For this review, take the finished solid that the model builds, in its own axes (mm). Coordinates: 2 decimals unless noted, no trailing zeros. Write each loop counter-clockwise with the first axis right and the second up, starting at its lowest first coordinate (ties: lowest second). Pieces come first, ordered by that corner, then holes. Notation, with made-up numbers: M 59,79.5 L 87,79.5 A19 ccw 87,109.5 Z; hole C 52,-28.75 d11. An arc over 180 degrees is marked long. One line per question, with ' | ' between items.
from build123d import *

# Parameters (mm, degrees)
SKETCH3_R           = 1.016
SKETCH3_R_2         = 0.75
BOSS_EXTRUDE1_DEPTH = 3


with BuildPart() as part:
    # Sketch3 → Boss-Extrude1 (new body)
    with BuildSketch(Plane.XY):
        with BuildLine():
            Line((9.525, -8.382), (41.275, -8.382))
            ThreePointArc((41.275, -8.382), (60.325, 10.668), (41.275, 29.718))
            Line((41.275, 29.718), (9.525, 29.718))
            ThreePointArc((9.525, 29.718), (-9.525, 10.668), (9.525, -8.382))
        make_face()
        with Locations((57.15, 10.668)):
            Circle(SKETCH3_R, mode=Mode.SUBTRACT)
        with Locations((-6.35, 10.668)):
            Circle(SKETCH3_R, mode=Mode.SUBTRACT)
        with Locations((2.032, 22.606)):
            Circle(SKETCH3_R_2, mode=Mode.SUBTRACT)
        with Locations((2.032, -1.27)):
            Circle(SKETCH3_R_2, mode=Mode.SUBTRACT)
        with Locations((49.022, -1.27)):
            Circle(SKETCH3_R_2, mode=Mode.SUBTRACT)
        with Locations((49.022, 22.606)):
            Circle(SKETCH3_R_2, mode=Mode.SUBTRACT)
        Polygon((18.5674, 24.638), (32.2326, 24.638), (32.2326, 21.59), (51.054, 21.59), (51.054, -0.254), (-0.254, -0.254), (-0.254, 21.59), (18.5674, 21.59), align=None, mode=Mode.SUBTRACT)
    extrude(amount=BOSS_EXTRUDE1_DEPTH)


solid = part.part
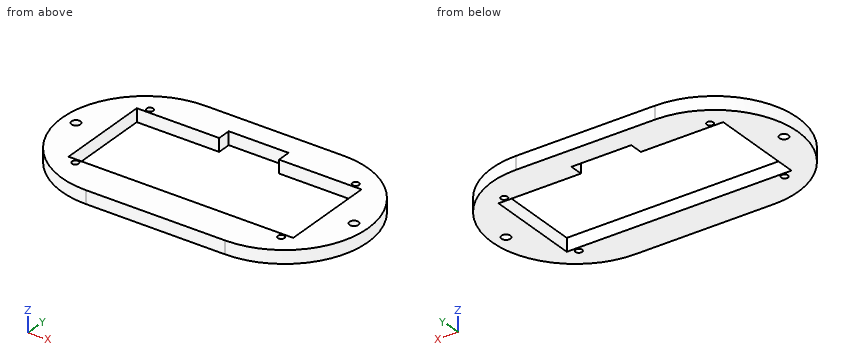
1. For line 1 along Y through (x, z) = (27.5, 2.3); line 2 along X through (y, z) = (10.5, 2.5); line 3 along Y through (x, z) = (2, 2.95), list the stretches that pass through material, from the lowest coordinate up.
Computed values:
line 1: y = -8.38 to -0.25, 24.64 to 29.72 | line 2: x = -9.52 to -7.35, -5.35 to -0.25, 51.05 to 56.15, 58.15 to 60.32 | line 3: y = -6.83 to -2.02, -0.52 to -0.25, 21.59 to 21.86, 23.36 to 28.17
2. Clearance check with flat-ended pins moving along their axes: P1, Ø1.5, axis at y = 6, z = 1, coming from the -X side; P2, Ø1.5, axis at y = 21, z = 1.5, coming from the +X side. State where each tip first meets the part, or that it passes through.
Computed values:
P1: stops at x = -9.12 | P2: stops at x = 57.74
3. Take a section at B-B on y = -1.27. State the section outline as (x, z) points, plus the area to 3 significant figures.
Computed values:
outline: M -5.32,0 L 1.28,0 L 1.28,3 L -5.32,3 Z; M 2.78,0 L 48.27,0 L 48.27,3 L 2.78,3 Z; M 49.77,0 L 56.12,0 L 56.12,3 L 49.77,3 Z | area: 175 mm2
4. Take a section at A-A on x = 25. State the section outline as (y, z) points, plus the area to 3 significant figures.
Computed values:
outline: M -8.38,0 L -0.25,0 L -0.25,3 L -8.38,3 Z; M 24.64,0 L 29.72,0 L 29.72,3 L 24.64,3 Z | area: 39.6 mm2
5. Take a section at C-C on x = 2. State the section outline as (y, z) points.
Computed values:
outline: M -6.83,0 L -2.02,0 L -2.02,3 L -6.83,3 Z; M -0.52,0 L -0.25,0 L -0.25,3 L -0.52,3 Z; M 21.59,0 L 21.86,0 L 21.86,3 L 21.59,3 Z; M 23.36,0 L 28.17,0 L 28.17,3 L 23.36,3 Z
6. Take a section at D-D on y = 9. State the section outline as (x, z) points, plus the area to 3 significant figures.
Computed values:
outline: M -9.45,0 L -0.25,0 L -0.25,3 L -9.45,3 Z; M 51.05,0 L 60.25,0 L 60.25,3 L 51.05,3 Z | area: 55.2 mm2
